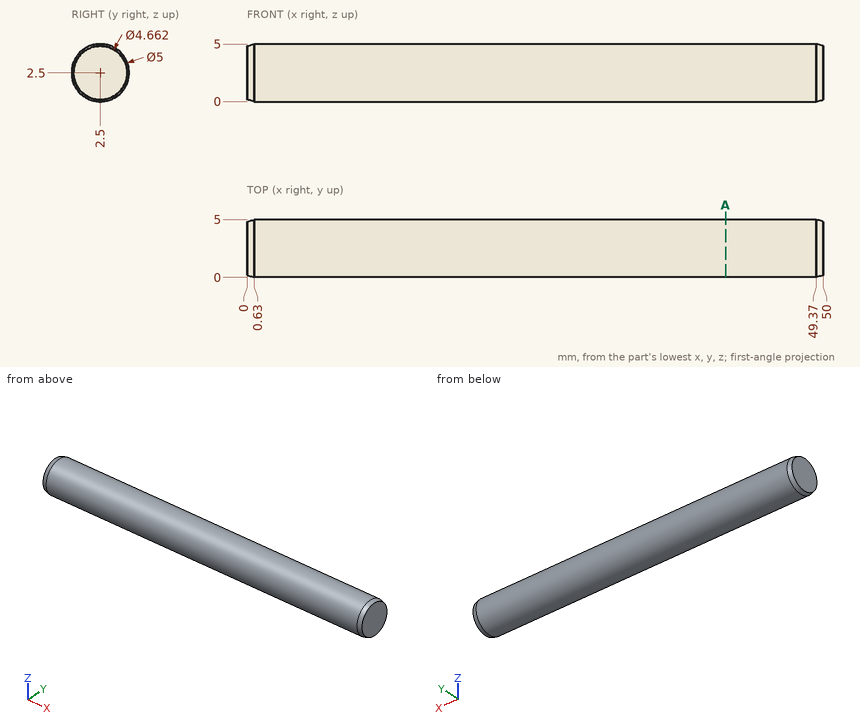
Design review of the part shown in the three views and the two pictorial views. Dimensions are in mm from the part's minimum x, y and z. Give positions to 0.01 mm unless a question says otherwise; leave off trailing zeros. Write each loop counter-clockwise with the first axis right and the second up, starting at its lowest first coordinate (ties: lowest second). Pieces come first, ordered by that corner, then holes. Notation, with made-up numbers: M -20,69.25 L 8,69.25 A20 cw 8,77.25 Z; hole C -13.5,-26.75 d3. An arc over 180 degrees is marked long. One line per question, with ' | ' between items. Start each with the question number.
Item 1: We need section A-A on x = 41.5. Write out the cut boundary in (y, z), plus the area to 3 significant figures.
Item 2: For pin 1 (1 mm diameter, centred on x = 43, z = 4, fed in from +Y); pin 2 (1 mm diameter, centred on x = 39, z = 1, fed in from -Y); pin 3 (1 mm diameter, centred on x = 34, z = 3.5, fed in from -Y), all flat-tipped, find the tip position at first contact; note any pin that passes through.
Item 3: Wall thickness on line 1 (Z direction, x = 16, y = 1); line 2 (Y direction, x = 36.5, z = 1.5); line 3 (Y direction, x = 4, z = 2.7): over which ranges is each line inside the solid? List them lowest first. Write a range as from..to.
Results found:
1) outline: C 2.5,2.5 d5 | area: 19.6 mm2
2) pin 1: stops at y = 4.79 | pin 2: stops at y = 0.21 | pin 3: stops at y = 0.05
3) line 1: z = 0.5..4.5 | line 2: y = 0.21..4.79 | line 3: y = 0.01..4.99
